Build history of the part. All positions in model axes, mm. A direction names the side the tool comes from. Round coordinates to 2 decimals unless told otherwise and drop trailing zeros. Order: outer loops, then holes, each group sorted by start corner. A loop starts at its lowest first (then second) coordinate and runs counter-clockwise, first axis right, second up. Notation, with made-up numbers: (63.25, 25) -> (86.25, 25) arc R11 ccw to (86.25, 43) -> close; hole circle Ø2 at (40, 4). An arc over 180 degrees is marked (long way). Use a Markdown table: item, result. Add a question column.
Item 1: Probe L1, parallel to X at y = 19, z = 0; L2, parallel to Y at x = -3.7, z = 0; L3, parallel to Y at x = -4, z = -2.25. List the from-to ranges inside material, lowest first.
Item 2: Two-plate mould, pull along Z, no slides. Class faces 1 (the face through (1.1, 22.86, -2.4)), 2 (the face through (-0.99, 9.26, -0.02)): released by +Z, released by -Z, zero draft, split by the parting line, or undercut.
Item 3: Slice it at B-B, the plane y = 6. Give the cut face in (x, z), plus the area to 3 significant figures.
Item 4: Slice it at A-A, the plane x = 1. Give the cut face in (y, z).
Item 5: 3-axis set-ups, long thin cutter, end or side, ignore diameter. For faces 3 (the face through (0, 8, 0)), 4 (the face through (-2.47, 16.42, -0.32)), 5 (the face through (-2, 0, 0)): which of +Z, -Z, +X, -X, +Y, -Y reach the whole face in a straight line?
Item 6: Slice it at C-C, the plane z = 0. Give the cut face in (x, y).
Item 7: Slice it at D-D, the plane y = 15.25. Give the cut face in (x, z).
Item 8: Pin check, flat tips, straight feed: pin 1 (3 mm diameter, centred on y = 4.76, z = 0, fed in from +X); pin 2 (1 mm diameter, centred on x = 1.5, z = -2.5, fed in from -Y); pin 3 (3 mm diameter, centred on x = 0, z = 0, fed in from +Y); pin 4 (1 mm diameter, centred on y = 7.5, z = 2.5, fed in from +X). Stop position of each tip, or through.
Autodesk Inventor part; units mm, degrees
ref_plane "YZ Plane" through (0, 0, 0) normal (1, 0, 0) x (0, 1, 0)
ref_plane "XZ Plane" through (0, 0, 0) normal (0, 1, 0) x (-1, 0, 0)
ref_plane "XY Plane" through (0, 0, 0) normal (0, 0, 1) x (1, 0, 0)
sketch "Sketch1" plane through (0, 0, 0) normal (0, 1, 0) x (-1, 0, 0)
  line L0 (0, 0) -> (4.7625, 0)
  line L1 (4.7625, 0) -> (4.7625, -2.7496)
  line L2 (4.7625, 0) -> (7.5121, 0) construction
  line L3 (4.7625, 0) -> (4.7625, 2.7496)
  line L4 (2.3813, 4.1244) -> (0, 5.4993)
  line L5 (2.3813, 4.1244) -> (4.7625, 2.7496)
  line L6 (-2.3813, 4.1244) -> (-4.7625, 2.7496)
  line L7 (-2.3813, 4.1244) -> (0, 5.4993)
  line L8 (-4.7625, 0) -> (-4.7625, -2.7496)
  line L9 (-4.7625, 0) -> (-4.7625, 2.7496)
  line L10 (-2.3812, -4.1244) -> (0, -5.4993)
  line L11 (-2.3812, -4.1244) -> (-4.7625, -2.7496)
  line L12 (2.3813, -4.1244) -> (4.7625, -2.7496)
  line L13 (2.3813, -4.1244) -> (0, -5.4993)
  line L14 (4.7625, 2.7496) -> (4.7625, -2.7496)
  line L15 (4.7625, -2.7496) -> (0, -5.4993)
  line L16 (0, -5.4993) -> (-4.7625, -2.7496)
  line L17 (-4.7625, -2.7496) -> (-4.7625, 2.7496)
  line L18 (-4.7625, 2.7496) -> (0, 5.4993)
  line L19 (4.7625, 2.7496) -> (0, 5.4993)
  dimension "d0" = 4.7625
  dimension "d1" = 90
  dimension "d4" = 360
extrude "Extrusion1" add sketch "Sketch1" along normal blind 22.86
sketch "Sketch2" plane through (0, 22.86, 0) normal (0, 1, 0) x (1, 0, 0)
  point P0 (0, 0)
  point P1 (0, 0)
hole "Hole1" at (0, 22.86, 0) direction (0, -1, 0) diameter 4.9784 depth 12.7 tip angle 118
sketch "Sketch3" plane through (0, 0, 0) normal (0, -1, 0) x (1, 0, 0)
  line L0 (0, 0) -> (9.2843, 0)
  line L1 (9.2843, 0) -> (9.2843, -7.4131)
  line L2 (9.2843, -7.4131) -> (0, -7.4131)
  line L3 (0, -7.4131) -> (0, 0)
  line L4 (9.2843, 0) -> (9.2843, 7.4131)
  line L5 (9.2843, 7.4131) -> (0, 7.4131)
  line L6 (0, 7.4131) -> (0, 0)
extrude "Extrusion2" cut sketch "Sketch3" against normal blind 12.7
sketch "Sketch5" plane through (0, 0, 5.4993) normal (1, 0, 0) x (0, 0, -1)
  line L0 (10.9985, 0) -> (10.9985, 12.7)
  line L1 (0, 0) -> (0, 12.7)
  line L2 (5.4993, 0) -> (5.4993, 4.7625)
  circle A0 centre (5.4993, 4.7625) radius 3.3782
  dimension "d17" = 4.7625
  dimension "d18" = 6.7564
hole "Hole2" at (0, 4.7625, 0) direction (-1, 0, 0) diameter 5.1054 end through all
properties part number "feet type 3 part 1 hexagon stock 10-32 hole" material "Aluminum 6061"
Check sheet entries:
| question | item | result |
|---|---|---|
| 1 | L1 | -4.76 to -2.49, 2.49 to 4.76 |
| 1 | L2 | 0 to 2.21, 7.32 to 22.86 |
| 1 | L3 | 0 to 3.56, 5.97 to 22.86 |
| 2 | face 1 | zero draft |
| 2 | face 2 | undercut |
| 3 | outline | (-4.76, -2.75) -> (-2.38, -4.12) -> (0, -5.5) -> (0, -2.23) -> (-4.76, -2.23) -> close; (-4.76, 2.23) -> (0, 2.23) -> (0, 5.5) -> (-2.38, 4.12) -> (-4.76, 2.75) -> close |
| 3 | area | 18.0 mm2 |
| 4 | outline | (12.7, -4.92) -> (22.86, -4.92) -> (22.86, -2.28) -> (12.7, -2.28) -> close; (12.7, 2.28) -> (22.86, 2.28) -> (22.86, 4.92) -> (12.7, 4.92) -> close |
| 5 | face 3 | +Z, -Z, +X, -Y |
| 5 | face 4 | +Y |
| 5 | face 5 | +Z, -Z, +X, -X, -Y |
| 6 | outline | (-4.76, 0) -> (0, 0) -> (0, 2.21) -> (-4.76, 2.21) -> close; (-4.76, 7.32) -> (0, 7.32) -> (0, 8.66) -> (-2.49, 10.16) -> (-2.49, 22.86) -> (-4.76, 22.86) -> close; (2.49, 12.7) -> (4.76, 12.7) -> (4.76, 22.86) -> (2.49, 22.86) -> close |
| 7 | outline | (-4.76, -2.75) -> (-2.38, -4.12) -> (0, -5.5) -> (2.38, -4.12) -> (4.76, -2.75) -> (4.76, 2.75) -> (2.38, 4.12) -> (0, 5.5) -> (-2.38, 4.12) -> (-4.76, 2.75) -> close; hole circle Ø4.98 at (0, 0) |
| 8 | pin 1 | through |
| 8 | pin 2 | y = 12.7 |
| 8 | pin 3 | y = 9.57 |
| 8 | pin 4 | x = 0 |
